from build123d import *

# Parameters (mm, degrees)
SKETCH_R           = 3.5
PAD_DEPTH          = 5
SKETCH001_W        = 4
SKETCH001_H        = 3
PAD001_DEPTH       = 7
POLARPATTERN_COUNT = 4


with BuildPart() as part:
    # Sketch → Pad (new body)
    with BuildSketch(Plane.XY):
        with BuildLine():
            Line((-9.5, 2), (-9.5, -2))
            Line((-9.5, -2), (-4.5, -2))
            ThreePointArc((-4.5, -2), (-3.482097, -3.482097), (-2, -4.5))
            Line((-2, -9.5), (-2, -4.5))
            Line((-2, -9.5), (2, -9.5))
            Line((2, -9.5), (2, -4.5))
            ThreePointArc((2, -4.5), (3.482097, -3.482097), (4.5, -2))
            Line((9.5, -2), (4.5, -2))
            Line((9.5, -2), (9.5, 2))
            Line((9.5, 2), (4.5, 2))
            ThreePointArc((4.5, 2), (3.482097, 3.482097), (2, 4.5))
            Line((2, 9.5), (2, 4.5))
            Line((2, 9.5), (-2, 9.5))
            Line((-2, 9.5), (-2, 4.5))
            ThreePointArc((-2, 4.5), (-3.482097, 3.482097), (-4.5, 2))
            Line((-9.5, 2), (-4.5, 2))
        make_face()
        Circle(SKETCH_R, mode=Mode.SUBTRACT)
    extrude(amount=-PAD_DEPTH)

    # Sketch001 → Pad001 (join)
    with BuildSketch(Plane.XY):
        with Locations((0, 8)):
            Rectangle(SKETCH001_W, SKETCH001_H)
    pad001 = extrude(amount=PAD001_DEPTH)

    # PolarPattern: Pad001 ×4 about axis
    polarpattern_axis = Axis((0, 0, 0), (0, 0, 1))
    for i in range(1, POLARPATTERN_COUNT):
        add(pad001.rotate(polarpattern_axis, i * 360 / POLARPATTERN_COUNT))


solid = part.part
Work out the finished part from the listing and answer in its coordinate system (mm). A direction names the side the tool comes from. Round coordinates to 2 decimals unless told otherwise and drop trailing zeros. Write each loop counter-clockwise with the first axis right and the second up, starting at its lowest first coordinate (ties: lowest second). Pieces come first, ordered by that corner, then holes. Notation, with made-up numbers: (32, 87.25) - (61, 87.25) arc R23 cw to (61, 96.25) - close; hole circle Ø7 at (51, 44.5). An arc over 180 degrees is marked (long way). Answer in a Markdown table with one row per item. Add a question column.
1. The mould has two halves that part along Y. Classify faces 1 (the cylindrical face through (-3.5, -3.464, -2.465)), 2 (the cylindrical face through (3.233, -1.341, -2.465)), 3 (the flat face through (0, 8, 7)): +Y half, -Y half, draft (parallel to the pull), parting line (faces both ways), or undercut.
2. For faces 4 (the flat face through (1.4, 3.4, 0)), 5 (the flat face through (0, 6.5, 3)), 6 (the flat face through (-6.5, 0, 3)), determine the directions among +Z, -Z, +X, -X, +Y, -Y from which every point of the face is accessible in a straight line to the end or side of a thin tool.
3. Find the intervals of material crossed by line 1 along X through (y, z) = (-0.75, 4.5); line 2 along Y through (x, z) = (0, -1.2); line 3 along Y through (x, z) = (8.75, -1.5), in increasing order. Write a range as from..to.
4. A cutting plane is placed at B-B, the plane z = 4.25. Determine the outline of the cut face in (x, y).
5. Given pin 1 (5.5 mm diameter, centred on x = -6, z = 3, fed in from +Y); pin 2 (2.5 mm diameter, centred on y = 8, z = 3, fed in from +X); pin 3 (10.5 mm diameter, centred on x = 1.5, y = 1, fed in from +Z); pin 4 (4 mm diameter, centred on y = 7.5, z = 1.5, fed in from -X), each flat-ended and moving along its own axis, determine where each tip first touches the part or whether it passes through.
6. A cutting plane is placed at D-D, the plane z = -1.5. Determine the outline of the cut face in (x, y).
7. A cutting plane is placed at A-A, the plane x = 0. Determine the outline of the cut face in (y, z).
Worked out:
| question | item | result |
|---|---|---|
| 1 | face 1 | -Y half |
| 1 | face 2 | undercut |
| 1 | face 3 | draft |
| 2 | face 4 | +Z |
| 2 | face 5 | +Z, +X, -X |
| 2 | face 6 | +Z, +Y, -Y |
| 3 | line 1 | -9.5..-6.5, 6.5..9.5 |
| 3 | line 2 | -9.5..-3.5, 3.5..9.5 |
| 3 | line 3 | -2..2 |
| 4 | outline | (-9.5, -2) - (-6.5, -2) - (-6.5, 2) - (-9.5, 2) - close; (-2, -9.5) - (2, -9.5) - (2, -6.5) - (-2, -6.5) - close; (-2, 6.5) - (2, 6.5) - (2, 9.5) - (-2, 9.5) - close; (6.5, -2) - (9.5, -2) - (9.5, 2) - (6.5, 2) - close |
| 5 | pin 1 | y = 2 |
| 5 | pin 2 | x = 2 |
| 5 | pin 3 | z = 7 |
| 5 | pin 4 | x = -2 |
| 6 | outline | (-9.5, -2) - (-4.5, -2) arc R4.92 ccw to (-2, -4.5) - (-2, -9.5) - (2, -9.5) - (2, -4.5) arc R4.92 ccw to (4.5, -2) - (9.5, -2) - (9.5, 2) - (4.5, 2) arc R4.92 ccw to (2, 4.5) - (2, 9.5) - (-2, 9.5) - (-2, 4.5) arc R4.92 ccw to (-4.5, 2) - (-9.5, 2) - close; hole circle Ø7 at (0, 0) |
| 7 | outline | (-9.5, -5) - (-3.5, -5) - (-3.5, 0) - (-6.5, 0) - (-6.5, 7) - (-9.5, 7) - close; (3.5, -5) - (9.5, -5) - (9.5, 7) - (6.5, 7) - (6.5, 0) - (3.5, 0) - close |
